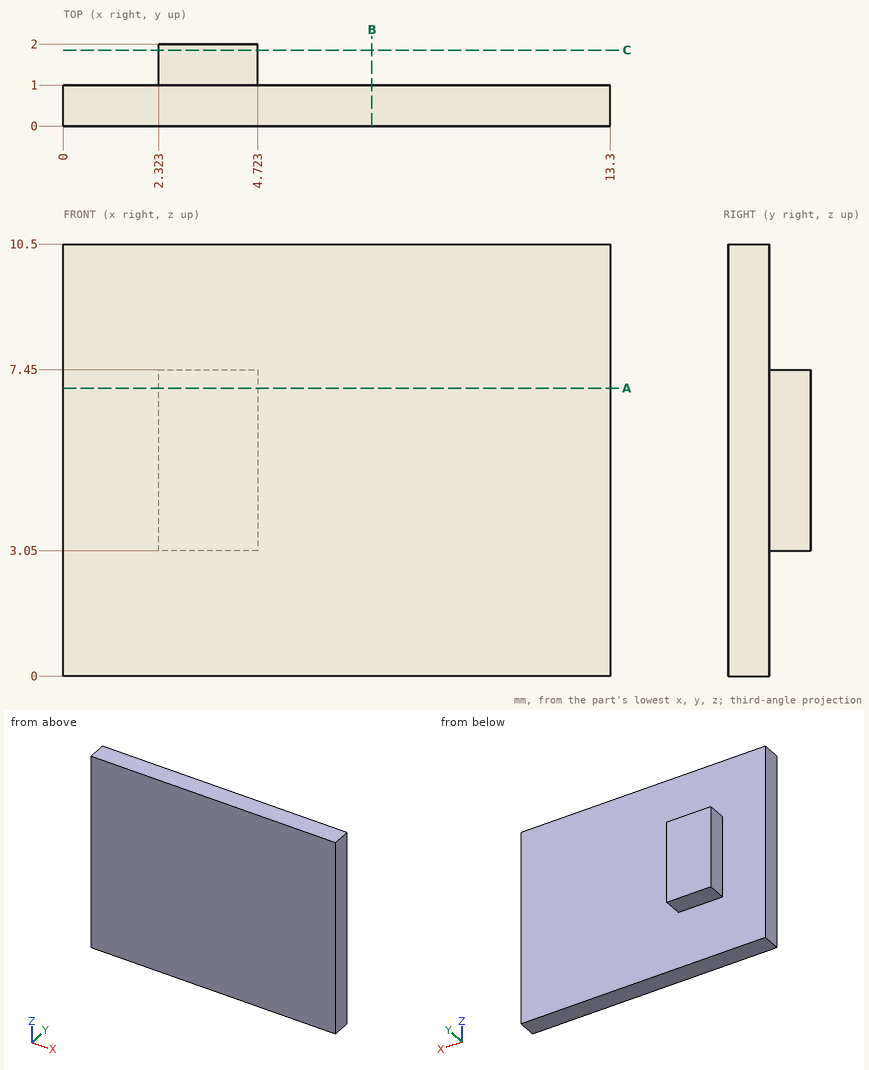
Job drawing, mm, ordinate dimensions from the low corner. One solid piece. Give positions to 0.01 mm unless a question says otherwise; leave off trailing zeros. Order: outer loops, then holes, each group sorted by start corner. A loop starts at its lowest first (then second) coordinate and runs counter-clockwise, first axis right, second up. Notation, with made-up numbers: M 21,61 L 44,61 A12 cw 44,70 Z; hole C 7,89 d5. An arc over 180 degrees is marked long. Put each result on its own line as item: value. Start each with the question number.
(1) Drill centre lines: L1, parallel to X at y = 1.7, z = 3.5; L2, parallel to Z at x = 3.25, y = 1.1; L3, parallel to Y at x = 12, z = 4.5. Where is each one in solid material? Low to high. Write a range as [from, to].
(2) Pin check, flat tip, straight feed: pin 1 Ø4 at (x, z) = (7.5, 8.5) entering from +Y. Stop position of the tip, or through.
(3) Band-saw the part on B-B on x = 7.5. Give the cut face in (y, z), then the cut area to 3 significant figures.
(4) Band-saw the part on A-A on z = 7. Give the cut face in (x, y), then the cut area to 3 significant figures.
(5) Band-saw the part on C-C on y = 1.85. Give the cut face in (x, z), then the cut area to 3 significant figures.
Results below:
1. L1: x = [2.32, 4.72]
1. L2: z = [3.05, 7.45]
1. L3: y = [0, 1]
2. pin 1: stops at y = 1
3. outline: M 0,0 L 1,0 L 1,10.5 L 0,10.5 Z
3. area: 10.5 mm2
4. outline: M 0,0 L 13.3,0 L 13.3,1 L 4.72,1 L 4.72,2 L 2.32,2 L 2.32,1 L 0,1 Z
4. area: 15.7 mm2
5. outline: M 2.32,3.05 L 4.72,3.05 L 4.72,7.45 L 2.32,7.45 Z
5. area: 10.6 mm2
